Source: three-view drawing plus pictorial views. Frame: mm from the lowest corner of the part. A direction names the side the tool comes from. Give positions to 0.01 mm unless a question says otherwise; leave off trailing zeros. Write each loop counter-clockwise with the first axis right and the second up, starting at its lowest first coordinate (ties: lowest second). Pieces come first, ordered by that corner, then holes. Notation, with made-up numbers: M -16,0.25 L 10,0.25 A10 ccw 10,8.25 Z; hole C 46.5,17.5 d11. An arc over 180 degrees is marked long. Return JSON: item names as keys, results as strings.
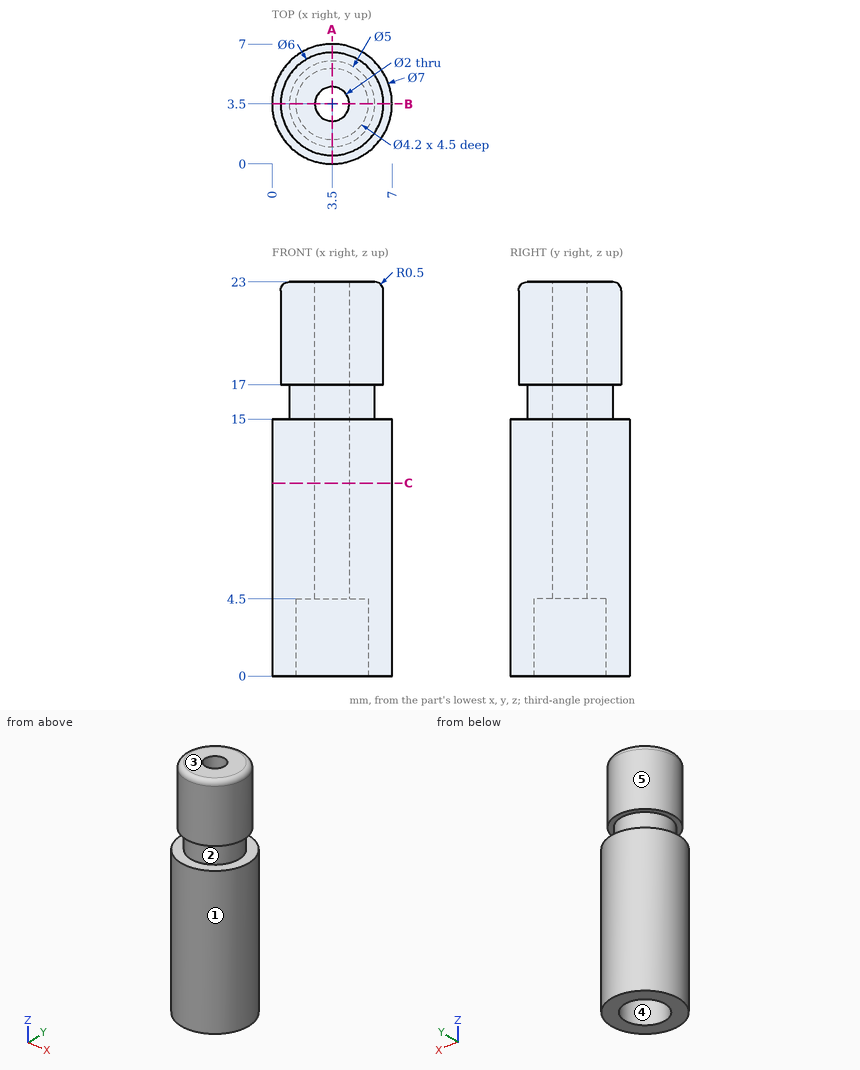
1) Cut plane A-A, the plane x = 3.5. Return the cut outline in (y, z), then the cut area to 3 significant figures.
Numbers:
{"outline": "M 0,0 L 1.4,0 L 1.4,4.5 L 2.5,4.5 L 2.5,23 L 1,23 A0.5 ccw 0.5,22.5 L 0.5,17 L 1,17 L 1,15 L 0,15 Z; M 4.5,4.5 L 5.6,4.5 L 5.6,0 L 7,0 L 7,15 L 6,15 L 6,17 L 6.5,17 L 6.5,22.5 A0.5 ccw 6,23 L 4.5,23 Z", "area": "95.0 mm²"}
2) Line query: line 1 (Y direction, x = 3.5, z = 15.5); line 2 (Y direction, x = 3.5, z = 17.5); line 3 (Z direction, x = 3, y = 2.5). Output: solid intervals per line, ascending. Write a range as [from, to].
Numbers:
{"line 1": "y = [1, 2.5], [4.5, 6]", "line 2": "y = [0.5, 2.5], [4.5, 6.5]", "line 3": "z = [4.5, 23]"}
3) Set-up query: the marked faces 1 and 2. Return all of +Z, -Z, +X, -X, +Y, -Y with unobstructed straight access to the full face (end or side cutting, diameter ignored); none if empty.
Numbers:
{"face 1": "+Z, -Z", "face 2": "none"}
4) Draft query along Y for the marked faces 3, 4 and 5. Return one class per face: released by +Y, released by -Y, zero draft, split by the parting line, or undercut.
Numbers:
{"face 3": "zero draft", "face 4": "undercut", "face 5": "split by the parting line"}
5) Cut plane C-C, the plane z = 11.25. Return the cut outline in (x, y), then the cut area to 3 significant figures.
Numbers:
{"outline": "C 3.5,3.5 d7; hole C 3.5,3.5 d2", "area": "35.3 mm²"}
6) Contact query for flat-ended pins moving along their axis: pin 1 Ø2.5 at (x, y) = (3.5, 3.5) entering from -Z; pin 2 Ø3 at (x, y) = (4.5, 4) entering from -Z; pin 3 Ø1 at (x, z) = (0.5, 10.5) entering from -Y. Output: stop coordinate, or through.
Numbers:
{"pin 1": "stops at z = 4.5", "pin 2": "stops at z = 0", "pin 3": "stops at y = 1.05"}
